```python
from build123d import *

# Parameters (mm, degrees)
F1_DEPTH = 7
F2_R     = 2
F3_R     = 0.8678369572
F4_SIZE  = 1.99999
F5_SIZE  = 1.99999


# Not quite as in the source:
# - a fillet or chamfer is up to 0.001 mm smaller than in the source, because OpenCascade refuses the exact size


with BuildPart() as f1:
    # F0 (on Top) → F1 (new body)
    with BuildSketch(Plane.XY):
        Polygon((9.1365975469, 13.0565894232), (-0.1652448664, 13.0565894232), (-9.5275098884, 13.0565894232), (-15.4519321666, -5.5724489729), (-0.1296436349, -16.7047432175), (15.0836615604, -5.6335964123), align=None)
        with BuildLine():
            ThreePointArc((-0.1630055447, 11.0487976356), (7.7556846484, 7.87095011), (11.05, 0))
            ThreePointArc((11.05, 0), (-7.7556846484, -7.87095011), (-0.1630055447, 11.0487976356))
        make_face(mode=Mode.SUBTRACT)
        Polygon((-9.5275098884, 13.0565894232), (-0.1652448664, 13.0565894232), (-0.1682447051, 15.7462661459), (-5.5240840498, 15.7462661459), (-0.1869622706, 32.5285686018), (-0.1979640721, 42.3928620705), align=None)
        Polygon((-0.1682447051, 15.7462661459), (-0.1652448664, 13.0565894232), (9.1365975469, 13.0565894232), (-0.1979640721, 42.3928620705), (-0.1869622706, 32.5285686018), (5.1325563495, 15.7462661459), align=None)
        Polygon((-15.4519321666, -5.5724489729), (-9.5275098884, 13.0565894232), (-41.0926038108, 13.0565894232), align=None)
        Polygon((-16.6826248751, -0.3878522951), (-30.9942816534, 9.8740688149), (-13.3895418888, 9.7472149984), align=None, mode=Mode.SUBTRACT)
        Polygon((40.7665927214, 13.0565894232), (9.1365975469, 13.0565894232), (15.0836615604, -5.6335964123), align=None)
        Polygon((13.2685531756, 10.1195799691), (30.8787326155, 10.2296921864), (16.561636162, -0.0154873244), align=None, mode=Mode.SUBTRACT)
        Polygon((-0.1296436349, -16.7047432175), (-15.4519321666, -5.5724489729), (-24.67217675, -34.5650295656), align=None)
        Polygon((-4.7863451446, -15.9859720469), (-18.9685572481, -26.4260584669), (-13.4077483305, -9.7221559812), align=None, mode=Mode.SUBTRACT)
        Polygon((24.2402355164, -34.4104968233), (15.0836615604, -5.6335964123), (-0.1296436349, -16.7047432175), align=None)
        Polygon((13.3053196858, -9.8071458261), (18.8518873485, -26.5213951891), (4.6839164999, -16.0709618918), align=None, mode=Mode.SUBTRACT)
    extrude(amount=F1_DEPTH)

    # F2
    f2_edges = [f1.edges().sort_by_distance(p)[0] for p in [
        (-0.197964, 42.392862, 3.5),
        (40.766593, 13.056589, 3.5),
        (24.240236, -34.410497, 3.5),
        (-24.672177, -34.56503, 3.5),
        (-41.092604, 13.056589, 3.5),
    ]]
    fillet(f2_edges, radius=F2_R)

    # F3
    f3_edges = [f1.edges().sort_by_distance(p)[0] for p in [
        (-18.968557, -26.426058, 3.5),
        (-30.994282, 9.874069, 3.5),
        (18.851887, -26.521395, 3.5),
        (30.878733, 10.229692, 3.5),
        (-0.186962, 32.528569, 3.5),
    ]]
    fillet(f3_edges, radius=F3_R)

    # F4 (size 2 in the source; OpenCascade refuses exactly that, so slightly less here)
    f4_edges = [f1.edges().sort_by_distance(p)[0] for p in [
        (-22.232373, 13.056589, 7),
        (-5.815451, 24.728966, 7),
        (-0.197607, 37.795214, 7),
        (5.422496, 24.729114, 7),
        (21.877967, 13.056589, 7),
        (36.521209, 11.675361, 7),
        (25.439911, 1.902936, 7),
        (18.738348, -17.119392, 7),
        (21.65782, -30.833222, 7),
        (9.590987, -23.767195, 7),
        (-9.935411, -23.840674, 7),
        (-19.137937, -17.162901, 7),
        (-25.78237, 1.933053, 7),
        (-36.83935, 11.674623, 7),
    ]]
    chamfer(f4_edges, length=F4_SIZE)

    # F5 (size 2 in the source; OpenCascade refuses exactly that, so slightly less here)
    f5_edges = [f1.edges().sort_by_distance(p)[0] for p in [
        (21.877967, 13.056589, 0),
        (5.422496, 24.729114, 0),
        (-5.815451, 24.728966, 0),
        (-22.232373, 13.056589, 0),
        (-25.78237, 1.933053, 0),
        (-19.137937, -17.162901, 0),
        (-9.935411, -23.840674, 0),
        (9.590987, -23.767195, 0),
        (25.439911, 1.902936, 0),
        (18.738348, -17.119392, 0),
        (-36.83935, 11.674623, 0),
        (-0.197607, 37.795214, 0),
        (36.521209, 11.675361, 0),
        (21.65782, -30.833222, 0),
        (-22.08788, -30.981637, 0),
    ]]
    chamfer(f5_edges, length=F5_SIZE)


solid = f1.part
```
CAD build for the part. Positions are in the model's coordinates, mm. A direction names the side the tool comes from. Coordinates: 2 decimals unless noted, no trailing zeros. Write each loop counter-clockwise with the first axis right and the second up, starting at its lowest first coordinate (ties: lowest second). Pieces come first, ordered by that corner, then holes.
(1) 3-axis set-ups, long thin cutter, end or side, ignore diameter. For faces 1 (the face through (24.107, 2.187, 6.014)), 2 (the face through (-10.073, -22.721, 1.014)), 3 (the face through (10.752, -20.547, 3.451)): which of +Z, -Z, +X, -X, +Y, -Y reach the whole face in a straight line?
(2) Two-plate mould, pull along X, no slides. Class faces 4 (the face through (-11, 3, 0)), 5 (the face through (-0.184, 36.559, 6.236)), 6 (the face through (-5.763, 24.892, 3.479)), 7 (the face through (8.934, -12.983, 3.451)): +X half, -X half, draft (parallel to the pull), parting line (faces both ways), or undercut.
(3) Cut at B-B, the plane x = -25. List the corners of the cut face in (y, z).
(4) Cut at C-C, the plane z = 3.5. Count the separate pieces of the cut face and the enclosed holes in it, and give its area (3 significant figures).
(5) Drill centre lines: probe 1 along Y at (x, z) = (0, 2.5); probe 2 along X at (y, z) = (-24, 1.75); probe 3 along X at (y, z) = (-23.5, 4.75). Where is each one in solid material? Low to high.
(6) Cut at A-A, the plane y = -1.5. List the corners of the cut face in (x, z), and give its area (3 significant figures).
(7) Flat gauge pins, fed straight in: pin 1 (0.9 mm diameter, centred on x = -17, z = 4, fed in from +Y); pin 2 (3 mm diameter, centred on y = 29.5, z = 5.5, fed in from +X); pin 3 (2 mm diameter, centred on y = -8.5, z = 0.5, fed in from +X); pin 4 (13.5 mm diameter, centred on x = 0, y = 0, fed in from +Z). Where does each tip first touch, or does it go through?
Geometry says:
1. face 1: +Z, +X
1. face 2: -Z, -Y
1. face 3: +Z, -Z
2. face 4: draft
2. face 5: parting line
2. face 6: -X half
2. face 7: undercut
3. outline: (1.36, 2) - (3.84, 0) - (5.58, 0) - (5.58, 7) - (3.84, 7) - (1.36, 5) - close; (9.83, 0) - (11.06, 0) - (13.06, 2) - (13.06, 5) - (11.06, 7) - (9.83, 7) - close
4. separate pieces: 1
4. enclosed holes: 6
4. area: 1,170 mm2
5. probe 1: y = -16.8 to -11.05, 11.05 to 15.75, 30.51 to 37.79
5. probe 2: x = -21.05 to -18.14, -15.67 to -10.58, 10.34 to 15.43, 18.01 to 20.67
5. probe 3: x = -21.15 to -17.99, -14.99 to -9.47, 9.22 to 14.76, 17.85 to 20.77
6. outline: (-21.06, 2) - (-17.65, 0) - (-10.95, 0) - (-10.95, 7) - (-17.65, 7) - (-21.06, 5) - close; (10.95, 0) - (17.36, 0) - (20.76, 2) - (20.76, 5) - (17.36, 7) - (10.95, 7) - close
6. area: 126 mm2
7. pin 1: stops at y = 13.06
7. pin 2: stops at x = 4.35
7. pin 3: stops at x = 15.52
7. pin 4: passes through
